```python
from build123d import *

# Parameters (mm, degrees)
SKETCH2_R           = 7
SKETCH2_R_2         = 2.125
BOSS_EXTRUDE2_DEPTH = 3
SKETCH3_W           = 118.4
SKETCH3_H           = 12.75
CUT_EXTRUDE1_DEPTH  = 338.231374578
SKETCH5_R           = 2.625
SKETCH5_R_2         = 4.075
SKETCH5_R_3         = 1.25
SKETCH5_R_4         = 1.625
SKETCH5_R_5         = 7
SKETCH5_W           = 6
SKETCH5_H           = 154
CUT_EXTRUDE2_DEPTH  = 338.231374578


with BuildPart() as part:
    # Sketch2 → Boss-Extrude2 (new body)
    with BuildSketch(Plane.XY):
        with BuildLine():
            Line((25.03035901, 0), (111.286489227, 49.8))
            ThreePointArc((111.286489227, 49.8), (152.858332199, 69.766604349), (181.6, 33.7))
            Line((181.6, 33.7), (181.6, 0))
            Line((181.6, 0), (300, 0))
            Line((300, 0), (300, 145))
            Line((300, 145), (38, 145))
            Line((38, 145), (38, 154))
            Line((38, 154), (19, 154))
            Line((19, 154), (0, 154))
            Line((0, 154), (0, 0))
            Line((0, 0), (25.03035901, 0))
        make_face()
        with Locations((19, 135)):
            Circle(SKETCH2_R, mode=Mode.SUBTRACT)
        with Locations((14, 149.5)):
            Circle(SKETCH2_R_2, mode=Mode.SUBTRACT)
        with Locations(Location((24, 149.5, 0), (0, 0, 180))):
            Circle(SKETCH2_R_2, mode=Mode.SUBTRACT)
        with Locations((24, 100.5)):
            Circle(SKETCH2_R_2, mode=Mode.SUBTRACT)
        with Locations((14, 100.5)):
            Circle(SKETCH2_R_2, mode=Mode.SUBTRACT)
    extrude(amount=BOSS_EXTRUDE2_DEPTH)

    # Sketch3 → Cut-Extrude1 (cut, through all)
    with BuildSketch(Plane.XY.offset(3)):
        with Locations((240.8, 6.375)):
            Rectangle(SKETCH3_W, SKETCH3_H)
    extrude(amount=-CUT_EXTRUDE1_DEPTH, mode=Mode.SUBTRACT)

    # Sketch5 → Cut-Extrude2 (cut, through all)
    with BuildSketch(Plane.XY.offset(3)):
        with Locations((254.98, 25.75)):
            Circle(SKETCH5_R)
        with Locations((234.98, 25.75)):
            Circle(SKETCH5_R)
        with Locations((288, 130)):
            Circle(SKETCH5_R_2)
        with Locations((288, 138.75)):
            Circle(SKETCH5_R_3)
        with Locations((288, 110.95)):
            Circle(SKETCH5_R_3)
        with Locations((285.78, 62.92)):
            Circle(SKETCH5_R_4)
        with Locations((181.6, 72.03)):
            Circle(SKETCH5_R_4)
        with Locations((52.23, 24.91)):
            Circle(SKETCH5_R_4)
        with Locations((112.84, 59.93)):
            Circle(SKETCH5_R_4)
        with Locations((266.895, 135.995)):
            Circle(SKETCH5_R_4)
        with Locations((128.895, 135.995)):
            Circle(SKETCH5_R_4)
        with Locations((214.98, 34.75)):
            Circle(SKETCH5_R_5)
        with Locations((3, 77)):
            Rectangle(SKETCH5_W, SKETCH5_H)
    extrude(amount=-CUT_EXTRUDE2_DEPTH, mode=Mode.SUBTRACT)


solid = part.part
```
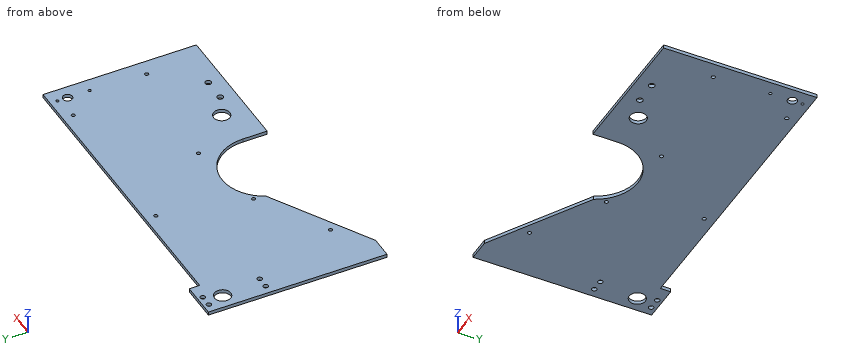
Part model, mm, in its own coordinate system. Round coordinates to 2 decimals unless told otherwise and drop trailing zeros. Write each loop counter-clockwise with the first axis right and the second up, starting at its lowest first coordinate (ties: lowest second). Pieces come first, ordered by that corner, then holes. Notation, with made-up numbers: M -0.75,45 L 6.25,45 A18 cw 6.25,50 Z; hole C -3,19.25 d9. An arc over 180 degrees is marked long. Answer as CSV lines item,"result". Start each with the question number.
1) Band-saw the part on A-A (z = 0.45). Count the separate pieces of the cut face and the enclosed holes in it, then the cut area to 3 significant figures.
2) Drill centre lines: L1, parallel to Y at x = 288, z = 1.2 (3 decimals); L2, parallel to X at y = 149.5, z = 1.45 (3 decimals); L3, parallel to X at y = 35, z = 0.8. Where is each one in solid material? Low to high.
3) Band-saw the part on B-B (x = 100.5). List the corners of the cut face in (y, z), then the cut area to 3 significant figures.
4) Drop flat-ended pins along their axis: pin 1 (6 mm diameter, centred on x = 254.98, y = 25.75, fed in from +Z); pin 2 (0.9 mm diameter, centred on x = 122, z = 1, fed in from +Y); pin 3 (1 mm diameter, centred on x = 82.5, z = 2.5, fed in from -Y). Give the stop position or say it passes through.
Worked out:
1,separate pieces,"1"
1,enclosed holes,"17"
1,area,"34,300 mm²"
2,L1,"12.75 to 109.7, 112.2 to 125.925, 134.075 to 137.5, 140 to 145"
2,L2,"6 to 11.875, 16.125 to 21.875, 26.125 to 38"
2,L3,"6 to 85.65, 181.58 to 207.98, 221.98 to 300"
3,outline,"M 43.57,0 L 145,0 L 145,3 L 43.57,3 Z"
3,area,"304 mm²"
4,pin 1,"z = 3"
4,pin 2,"y = 145"
4,pin 3,"y = 32.89"
